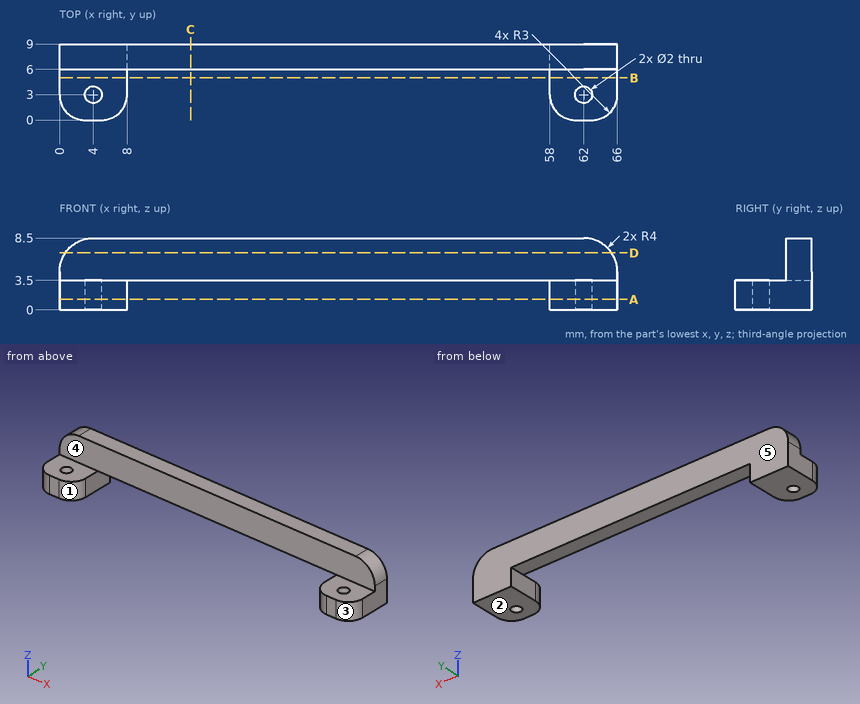
Verification items for this drawing (mm, ordinates from the low corner). A direction names the side the tool comes from. Coordinates: 2 decimals unless noted, no trailing zeros. Write each loop counter-clockwise with the first axis right and the second up, starting at its lowest first coordinate (ties: lowest second). Pieces come first, ordered by that corner, then holes. Notation, with made-up numbers: M 59.5,2 L 70.5,2 A27 cw 70.5,18 Z; hole C 81,-30 d3. An arc over 180 degrees is marked long. Use CSV: the item, a comma, the result in double quotes.
Q1. Set-up check for the marked faces 4 and 5: record each of +Z, -Z, +X, -X, +Y, -Y from which the full face is reachable in a straight line by a thin tool's end or side.
Computed values:
face 4,"+Z, +X, -X, -Y"
face 5,"+Z, -Z, +X, -X, +Y"
Q2. Section check D-D, the plane z = 6.75. Enter the section's corners in (x, y), and give its area (3 significant figures).
Computed values:
outline,"M 0.69,6 L 65.31,6 L 65.31,9 L 0.69,9 Z"
area,"194 mm²"
Q3. Section check B-B, the plane y = 5. Enter the section's corners in (x, z).
Computed values:
outline,"M 0,0 L 8,0 L 8,3.5 L 0,3.5 Z; M 58,0 L 66,0 L 66,3.5 L 58,3.5 Z"
Q4. Section check A-A, the plane z = 1.25. Enter the section's corners in (x, y).
Computed values:
outline,"M 0,3 A3 ccw 3,0 L 5,0 A3 ccw 8,3 L 8,9 L 0,9 Z; M 58,3 A3 ccw 61,0 L 63,0 A3 ccw 66,3 L 66,9 L 58,9 Z; hole C 4,3 d2; hole C 62,3 d2"
Q5. Mould release check, pull along X, two halves, no side actions. Record for the marked faces 1, 2 and 3: pulls with the +X half, pulls with the -X half, needs draft (parallel to the pull), parting line crosses it, or undercut.
Computed values:
face 1,"undercut"
face 2,"needs draft"
face 3,"pulls with the +X half"
Q6. Section check C-C, the plane x = 15.5. Enter the section's corners in (y, z), and give its area (3 significant figures).
Computed values:
outline,"M 6,3.5 L 9,3.5 L 9,8.5 L 6,8.5 Z"
area,"15.0 mm²"
Q7. Thickness scan on line 1 along X through (y, z) = (3, 2.6); line 2 along Y through (x, z) = (4, 2.1); line 3 along X through (y, z) = (5, 2.5). Record the ranges inside material, lowest first. Write a range as [from, to].
Computed values:
line 1,"[0, 3], [5, 8], [58, 61], [63, 66]"
line 2,"[0, 2], [4, 9]"
line 3,"[0, 8], [58, 66]"
Q8. Go/stop test with flat-tipped pins: P1, Ø4, axis at x = 37, z = 3, coming from the -Y side; P2, Ø2.5, axis at x = 4, y = 3, coming from the -Z side; P3, Ø2.5, axis at x = 41.5, y = 7.5, coming from the -Z side. Record where each tip stops, or that it passes through.
Computed values:
P1,"y = 6"
P2,"z = 0"
P3,"z = 3.5"
